Geometry check sheet. Reference: the model listing, model coordinates, mm. Give positions to 0.01 mm unless a question says otherwise; leave off trailing zeros. Order: outer loops, then holes, each group sorted by start corner. A loop starts at its lowest first (then second) coordinate and runs counter-clockwise, first axis right, second up. Notation, with made-up numbers: M 26.25,28 L 63.25,28 A9 cw 63.25,35 Z; hole C -8,-1 d5. An arc over 180 degrees is marked long. Answer as CSV lines item,"result". Start each with the question number.
Q1. Section check C-C, the plane y = -42. Record the boundary of the cut face in (x, z), then the cut area to 3 significant figures.
Q2. Section check D-D, the plane x = 22. Record the boundary of the cut face in (y, z), then the cut area to 3 significant figures.
Q3. Section check A-A, the plane x = -42.5. Record the boundary of the cut face in (y, z), then the cut area to 3 significant figures.
Q4. Section check B-B, the plane z = 5. Record the boundary of the cut face in (x, y), then the cut area to 3 significant figures.
Q5. Go/stop test with flat-tipped pins: pin 1 (1.5 mm diameter, centred on x = 9, z = 9, fed in from +Y); pin 2 (6.5 mm diameter, centred on x = -13.34, y = -22.82, fed in from +Z); pin 3 (5 mm diameter, centred on x = 14, z = 2, fed in from +Y). Record where each tip stops, or that it passes through.
Q6. Mould release check, pull along X, two halves, no side actions. Record for faces 1 (the flat face through (-50, 34.376, 5)), 2 (the flat face through (8.307, 27.936, 4.955)), 3 (the cylindrical face through (-12.821, -18.858, 4.955)): +X half, -X half, draft (parallel to the pull), parting line (faces both ways), or undercut.
Q7. Thickness scan on line 1 (X direction, y = -20, z = 7.5); line 2 (X direction, y = -19.5, z = 9); line 3 (Y direction, x = -17, z = 4.75). Record the ranges inside material, lowest first.
```python
from build123d import *

# Parameters (mm, degrees)
SKETCH1_W      = 122
SKETCH1_H      = 82.6
EXTRUDE1_DEPTH = 10.05
SKETCH2_R      = 4
EXTRUDE2_DEPTH = 11.05
EXTRUDE3_DEPTH = 11.05
FILLET1_R      = 10
FILLET2_R      = 20


with BuildPart() as part:
    # Sketch1 → Extrude1 (new body)
    with BuildSketch(Plane.XY):
        with Locations((-29.941398377, -6.923807929)):
            Rectangle(SKETCH1_W, SKETCH1_H)
    extrude(amount=EXTRUDE1_DEPTH)

    # Sketch2 → Extrude2 (cut, through all)
    with BuildSketch(Plane(origin=(0, 0, 0), x_dir=(-1, 0, 0), z_dir=(0, 0, -1))):
        with Locations((45.141398377, 8.976192071)):
            Circle(SKETCH2_R)
        with Locations((45.141398377, -22.823807929)):
            Circle(SKETCH2_R)
        with Locations((13.341398377, 8.976192071)):
            Circle(SKETCH2_R)
        with Locations((13.341398377, -22.823807929)):
            Circle(SKETCH2_R)
    extrude(amount=-EXTRUDE2_DEPTH, mode=Mode.SUBTRACT)

    # Sketch3 → Extrude3 (cut, through all)
    with BuildSketch(Plane(origin=(0, 0, 0), x_dir=(-1, 0, 0), z_dir=(0, 0, -1))):
        Polygon((4.941398377, 34.376192071), (-31.058601623, 16.876192071), (-39.457911359, 42.934117224), align=None)
        Polygon((-31.058601623, -30.723807929), (-39.457911359, -56.781733081), (4.941398377, -48.223807929), align=None)
    extrude(amount=-EXTRUDE3_DEPTH, mode=Mode.SUBTRACT)

    # Fillet1
    fillet1_edges = [part.edges().sort_by_distance(p)[0] for p in [
        (-4.941398377, 34.376192071, 5.025),
        (-4.941398377, -48.223807929, 5.025),
    ]]
    fillet(fillet1_edges, radius=FILLET1_R)

    # Fillet2
    fillet2_edges = [part.edges().sort_by_distance(p)[0] for p in [
        (31.058601623, 16.876192071, 5.025),
        (31.058601623, -30.723807929, 5.025),
    ]]
    fillet(fillet2_edges, radius=FILLET2_R)


solid = part.part
```
Answer block:
1,outline,"M -90.94,0 L 7.86,0 L 7.86,10.05 L -90.94,10.05 Z"
1,area,"993 mm2"
2,outline,"M -34.95,0 L 21.1,0 L 21.1,10.05 L -34.95,10.05 Z"
2,area,"563 mm2"
3,outline,"M -48.22,0 L -25.83,0 L -25.83,10.05 L -48.22,10.05 Z; M -19.82,0 L 5.97,0 L 5.97,10.05 L -19.82,10.05 Z; M 11.98,0 L 34.38,0 L 34.38,10.05 L 11.98,10.05 Z"
3,area,"709 mm2"
4,outline,"M -90.94,-48.22 L -7.24,-48.22 A10 ccw -2.87,-47.22 L 19.8,-36.2 A20 ccw 31.06,-18.21 L 31.06,4.36 A20 ccw 19.8,22.35 L -2.87,33.37 A10 ccw -7.24,34.38 L -90.94,34.38 Z; hole C -45.14,-22.82 d8; hole C -45.14,8.98 d8; hole C -13.34,-22.82 d8; hole C -13.34,8.98 d8"
4,area,"9,190 mm2"
5,pin 1,"stops at y = 27.96"
5,pin 2,"passes through"
5,pin 3,"stops at y = 26.38"
6,face 1,"draft"
6,face 2,"+X half"
6,face 3,"undercut"
7,line 1,"x = -90.94 to -47.97, -42.31 to -16.17, -10.51 to 30.98"
7,line 2,"x = -90.94 to -47.37, -42.92 to -15.57, -11.12 to 31.02"
7,line 3,"y = -48.22 to -24.44, -21.21 to 7.36, 10.59 to 34.38"
